CAD build for the part. Positions are in the model's coordinates, mm. A direction names the side the tool comes from. Coordinates: 2 decimals unless noted, no trailing zeros. Loops run counter-clockwise (first coordinate to the right, second up) from the corner with the lowest first, then second, coordinate; pieces in that order, holes last. Notation, with made-up numbers: M 66,5 L 89,5 A8 ccw 89,12 Z; hole C -31.5,56.25 d8. An arc over 180 degrees is marked long. Answer as a JSON object with one key per item and string values. Group by question number.
```python
from build123d import *

# Parameters (mm, degrees)
SKETCH2_W           = 20
SKETCH2_H           = 10
BOSS_EXTRUDE1_DEPTH = 2.5
FILLET1_R           = 5
SKETCH3_R           = 4.5
BOSS_EXTRUDE2_DEPTH = 4.4
FILLET2_R           = 2.5


with BuildPart() as part:
    # Sketch2 → Boss-Extrude1 (new body)
    with BuildSketch(Plane.XZ):
        with Locations((0, -40)):
            Rectangle(SKETCH2_W, SKETCH2_H)
    extrude(amount=BOSS_EXTRUDE1_DEPTH)

    # Fillet1
    fillet1_edges = [part.edges().sort_by_distance(p)[0] for p in [
        (-10, -1.25, -35),
        (-10, -1.25, -45),
        (10, -1.25, -45),
        (10, -1.25, -35),
    ]]
    fillet(fillet1_edges, radius=FILLET1_R - 0.0001)  # a hair under: the kernel refuses the full size

    # Sketch3 → Boss-Extrude2 (add)
    with BuildSketch(Plane.XZ.offset(2.5)):
        with Locations(Location((0, -40, 0), (0, 0, 270))):
            Circle(SKETCH3_R)
    extrude(amount=BOSS_EXTRUDE2_DEPTH)

    # Fillet2
    fillet2_edges = [part.edges().sort_by_distance(p)[0] for p in [
        (0, -6.9, -35.5),
    ]]
    fillet(fillet2_edges, radius=FILLET2_R)


solid = part.part
```
Item 1: Drill centre lines: L1, parallel to Y at x = 6.25, z = -37; L2, parallel to Y at x = 4, z = -41; L3, parallel to Z at x = -2.75, y = -3.25. Where is each one in solid material? Low to high. Write a range as from..to.
Item 2: Slice it at B-B, the plane x = -6.5. Write the cut outline in (y, z), then the cut area to 3 significant figures.
Item 3: Tool access for faces 1 (the cylindrical face through (1.352, -3.437, -44.292)), 2 (the cylindrical face through (-9, -1, -37)): list every direction of +Z, -Z, +X, -X, +Y, -Y with a clear straight run to the whole face (end or side of a thin tool).
Item 4: Pin check, flat tips, straight feed: pin 1 (3 mm diameter, centred on x = -6.5, z = -44, fed in from -Y); pin 2 (5 mm diameter, centred on x = -4, z = -37, fed in from -Y); pin 3 (3 mm diameter, centred on x = -8, y = -1, fed in from -Z). Stop position of each tip, or through.
Computed:
{
 "1": {"L1": "-2.5..0", "L2": "-5.72..0", "L3": "-43.56..-36.44"},
 "2": {"outline": "M -2.5,-44.77 L 0,-44.77 L 0,-35.23 L -2.5,-35.23 Z", "area": "23.8 mm2"},
 "3": {"face 1": "-Y", "face 2": "+Z, -X, +Y, -Y"},
 "4": {"pin 1": "y = -2.5", "pin 2": "y = -6.85", "pin 3": "z = -44.77"}
}
